CAD build for the part. Positions are in the model's coordinates, mm. A direction names the side the tool comes from. Coordinates: 2 decimals unless noted, no trailing zeros. Loops run counter-clockwise (first coordinate to the right, second up) from the corner with the lowest first, then second, coordinate; pieces in that order, holes last.
1) Saw through at C-C, the plane x = 57. Write the cut outline in (y, z) (3 decimals), and give its area (3 significant figures).
2) Two-plate mould, pull along Y, no slides. Class faces 3 (the flat face through (0, 0, 0)), 4 (the flat face through (38, 15.875, 0)), 5 (the cylindrical face through (62.39, -3.1, 0.69)): +Y half, -Y half, draft (parallel to the pull), parting line (faces both ways), or undercut.
3) Saw through at A-A, the plane y = 0. Write the cut outline in (x, z) (3 decimals), and give its area (3 significant figures).
4) Which spindle directions (+Z, -Z, +X, -X, +Y, -Y) get a long thin tool onto all of the face, cutting with end or side? Do faces 1 (the flat face through (38, 0, 15.875)), 2 (the flat face through (50.8, 0, 0)). Say none if no direction does.
5) Pin check, flat tips, straight feed: pin 1 Ø5 at (y, z) = (-1, 1) entering from +X; pin 2 Ø5.5 at (y, z) = (0, 0) entering from +X. Stop position of each tip, or through.
6) Wall check: line 1 along Y through (x, z) = (66, 0) (3 decimals); line 2 along Z through (x, y) = (59, 2) (3 decimals); line 3 along Z through (x, y) = (61, 1) (3 decimals). Give the ranges that are in metal, low to high.
```python
from build123d import *

# Parameters (mm, degrees)
SKETCH1_W           = 31.75
SKETCH1_H           = 31.75
BOSS_EXTRUDE1_DEPTH = 76.2
SKETCH2_R           = 3.175
CUT_EXTRUDE1_DEPTH  = 25.4
CHAMFER1_SIZE       = 2.54


with BuildPart() as part:
    # Sketch1 → Boss-Extrude1 (new body)
    with BuildSketch(Plane(origin=(0, 0, 0), x_dir=(0, 0, -1), z_dir=(1, 0, 0))):
        Rectangle(SKETCH1_W, SKETCH1_H)
    extrude(amount=BOSS_EXTRUDE1_DEPTH)

    # Sketch2 → Cut-Extrude1 (cut)
    with BuildSketch(Plane(origin=(76.2, 0, 0), x_dir=(0, 0, -1), z_dir=(1, 0, 0))):
        Circle(SKETCH2_R)
    extrude(amount=-CUT_EXTRUDE1_DEPTH, mode=Mode.SUBTRACT)

    # Chamfer1
    chamfer1_edges = [part.edges().sort_by_distance(p)[0] for p in [
        (76.2, 0, 3.175),
    ]]
    chamfer(chamfer1_edges, length=CHAMFER1_SIZE)


solid = part.part
```
Data:
1. outline: (-15.875, -15.875) - (15.875, -15.875) - (15.875, 15.875) - (-15.875, 15.875) - close; hole circle Ø6.35 at (0, 0)
1. area: 976 mm2
2. face 3: draft
2. face 4: +Y half
2. face 5: undercut
3. outline: (0, -15.875) - (76.2, -15.875) - (76.2, -5.715) - (73.66, -3.175) - (50.8, -3.175) - (50.8, 3.175) - (73.66, 3.175) - (76.2, 5.715) - (76.2, 15.875) - (0, 15.875) - close
3. area: 2,250 mm2
4. face 1: +Z, +X, -X, +Y, -Y
4. face 2: +X
5. pin 1: stops at x = 74.4
5. pin 2: stops at x = 50.8
6. line 1: y = -15.875 to -3.175, 3.175 to 15.875
6. line 2: z = -15.875 to -2.466, 2.466 to 15.875
6. line 3: z = -15.875 to -3.013, 3.013 to 15.875
